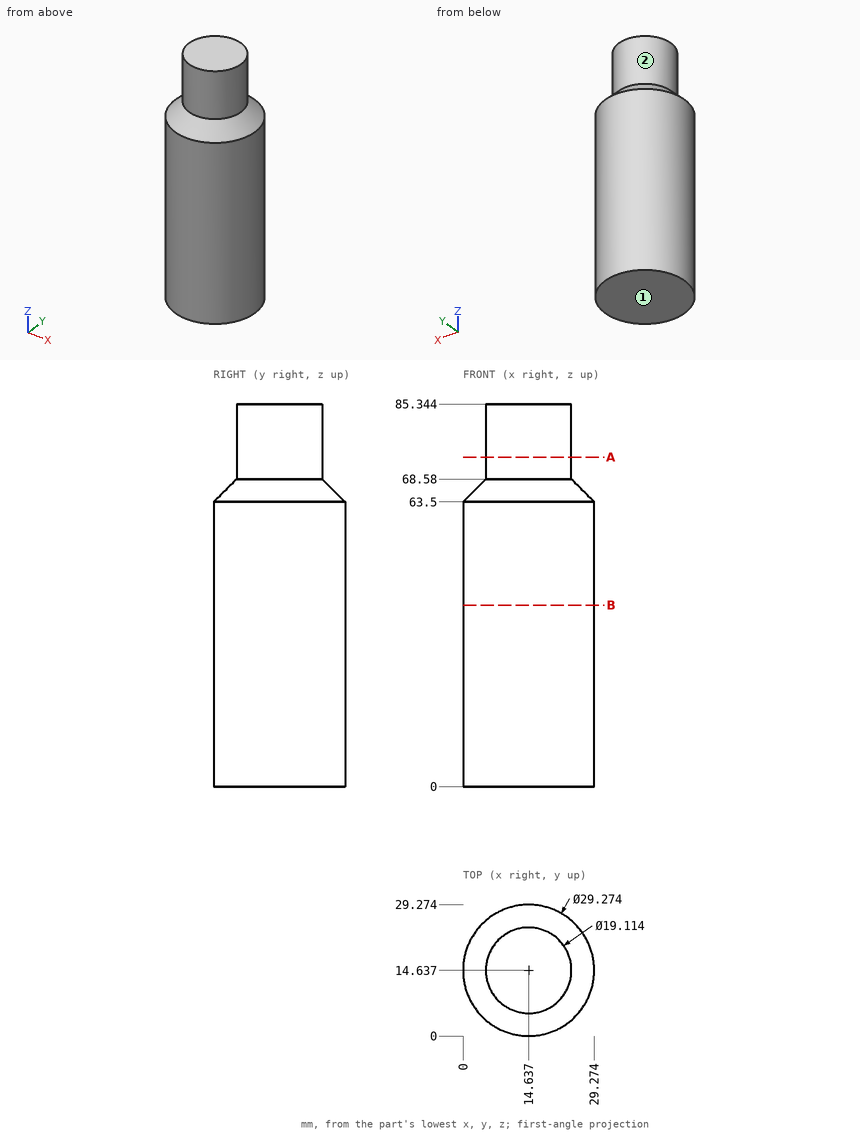
The drawing under review shows one solid part. Ordinate dimensions are in mm from its lowest x, y, z. A direction names the side the tool comes from. Round coordinates to 2 decimals unless told otherwise and drop trailing zeros. Write each loop counter-clockwise with the first axis right and the second up, starting at its lowest first coordinate (ties: lowest second). Pieces come first, ordered by that corner, then holes. Notation, with made-up numbers: (13.5, 58.25) - (27.5, 58.25) arc R32 ccw to (27.5, 92.25) - close; hole circle Ø2 at (-6, -1). An arc over 180 degrees is marked (long way). Use a Markdown table: item, result. Add a question column.
1. We need section A-A (z = 73.5). State the section outline as (x, y) points.
2. For the marked faces 1 and 2, list the 3-axis set-ups (+Z, -Z, +X, -X, +Y, -Y) from which the entire face can be reached by the end or side of a thin tool; tool diameter is ignored.
3. Clearance check with flat-ended pins moving along their axes: pin 1 (1 mm diameter, centred on y = 23.5, z = 18.5, fed in from -X); pin 2 (5 mm diameter, centred on x = 16.5, y = 9.5, fed in from -Z); pin 3 (10 mm diameter, centred on y = 9.5, z = 11.5, fed in from +X); pin 4 (5 mm diameter, centred on y = 25.5, z = 66.5, fed in from +X). State where each tip first meets the part, or that it passes through.
4. Wall thickness on probe 1 along X at (y, z) = (8, 57); probe 2 along X at (y, z) = (22.5, 4); probe 3 along Y at (x, z) = (14.25, 42.5): over which ranges is each line inside the solid? List them lowest first.
5. We need section B-B (z = 40.5). State the section outline as (x, y) points, then the cut area to 3 significant figures.
Output:
| question | item | result |
|---|---|---|
| 1 | outline | circle Ø19.11 at (14.64, 14.64) |
| 2 | face 1 | -Z, +X, -X, +Y, -Y |
| 2 | face 2 | +Z |
| 3 | pin 1 | stops at x = 2.62 |
| 3 | pin 2 | stops at z = 0 |
| 3 | pin 3 | stops at x = 29.27 |
| 3 | pin 4 | stops at x = 24.56 |
| 4 | probe 1 | x = 1.59 to 27.68 |
| 4 | probe 2 | x = 2.29 to 26.98 |
| 4 | probe 3 | y = 0.01 to 29.27 |
| 5 | outline | circle Ø29.27 at (14.64, 14.64) |
| 5 | area | 673 mm2 |
